```python
from build123d import *

# Parameters (mm, degrees)
F1_DEPTH = 5


with BuildPart() as f1:
    # F0 (on Right) → F1 (new body)
    with BuildSketch(Plane.YZ):
        with BuildLine():
            Line((-17.5, 52), (-22.5, 52))
            Line((-22.5, 52), (-22.5, 47))
            Line((-22.5, 47), (-23.8, 47))
            ThreePointArc((-23.8, 47), (-32.285281, 43.485281), (-35.8, 35))
            Line((-35.8, 35), (-35.8, 26))
            Line((-35.8, 26), (-34.8, 26))
            ThreePointArc((-34.8, 26), (-29.850253, 28.050253), (-27.8, 33))
            Line((-27.8, 33), (-27.8, 33.8))
            ThreePointArc((-27.8, 33.8), (-27.741421, 33.941421), (-27.6, 34))
            Line((-27.6, 34), (-22.7, 34))
            ThreePointArc((-22.7, 34), (-22.558579, 33.941421), (-22.5, 33.8))
            Line((-22.5, 33.8), (-22.5, -1))
            Line((-22.5, -1), (-23.8, -1))
            ThreePointArc((-23.8, -1), (-32.285281, -4.514719), (-35.8, -13))
            Line((-35.8, -13), (-35.8, -22))
            Line((-35.8, -22), (-34.8, -22))
            ThreePointArc((-34.8, -22), (-29.850253, -19.949747), (-27.8, -15))
            Line((-27.8, -15), (-27.8, -14.2))
            ThreePointArc((-27.8, -14.2), (-27.741421, -14.058579), (-27.6, -14))
            Line((-27.6, -14), (-22.7, -14))
            ThreePointArc((-22.7, -14), (-22.558579, -14.058579), (-22.5, -14.2))
            Line((-22.5, -14.2), (-22.5, -52))
            Line((-22.5, -52), (-17.5, -52))
            Line((-17.5, -52), (-17.5, -57))
            Line((-17.5, -57), (-7.5, -57))
            Line((-7.5, -57), (-7.5, -52))
            Line((-7.5, -52), (7.5, -52))
            Line((7.5, -52), (7.5, -57))
            Line((7.5, -57), (17.5, -57))
            Line((17.5, -57), (17.5, -52))
            Line((17.5, -52), (22.5, -52))
            Line((22.5, -52), (22.5, -45))
            Line((22.5, -45), (27.5, -45))
            Line((27.5, -45), (27.5, -27))
            Line((27.5, -27), (22.5, -27))
            Line((22.5, -27), (22.5, 27))
            Line((22.5, 27), (27.5, 27))
            Line((27.5, 27), (27.5, 45))
            Line((27.5, 45), (22.5, 45))
            Line((22.5, 45), (22.5, 52))
            Line((22.5, 52), (17.5, 52))
            Line((17.5, 52), (17.5, 57))
            Line((17.5, 57), (7.5, 57))
            Line((7.5, 57), (7.5, 52))
            Line((7.5, 52), (-7.5, 52))
            Line((-7.5, 52), (-7.5, 57))
            Line((-7.5, 57), (-17.5, 57))
            Line((-17.5, 57), (-17.5, 52))
        make_face()
    extrude(amount=F1_DEPTH)


solid = f1.part
```
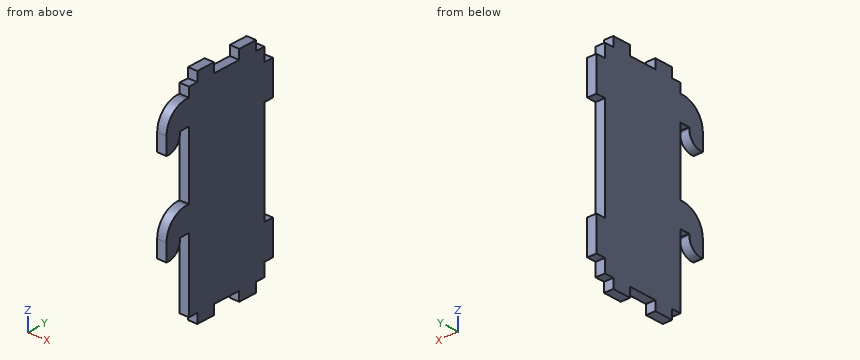
Work out the finished part from the listing and answer in its coordinate system (mm). Round coordinates to 2 decimals unless told otherwise and drop trailing zeros. Loops run counter-clockwise (first coordinate to the right, second up) from the corner with the lowest first, then second, coordinate; pieces in that order, holes last.
(1) Find the intervals of material crossed by L1, parallel to Y at x = 2.05, z = 52.5; L2, parallel to Z at x = 3.95, y = 3.5; L3, parallel to Y at x = 3.3, z = 3, in increasing order.
Computed values:
L1: y = -17.5 to -7.5, 7.5 to 17.5
L2: z = -52 to 52
L3: y = -22.5 to 22.5
(2) The part is cut by section C-C, the plane y = 4. Give the vertices of the cut face in (x, z).
Computed values:
outline: (0, -52) - (5, -52) - (5, 52) - (0, 52) - close
(3) Each of these flat-tipped pins is pushed along its axis until it touches: P1, Ø2.5, axis at x = 2, y = 24, coming from the +Z side; P2, Ø0.7, axis at x = 3.5, y = -23, coming from the +Z side; P3, Ø2.5, axis at x = 3.5, y = -21, coming from the -Z side. Where does it stop, or does it pass through?
Computed values:
P1: stops at z = 45
P2: stops at z = 47
P3: stops at z = -52
(4) The part is cut by section B-B, the plane z = -31. Give the vertices of the cut face in (x, y), and give its area (3 significant figures).
Computed values:
outline: (0, -22.5) - (5, -22.5) - (5, 27.5) - (0, 27.5) - close
area: 250 mm2
(5) The part is cut by section A-A, the plane y = -31.5. Give the vertices of the cut face in (x, z).
Computed values:
outline: (0, -21.17) - (5, -21.17) - (5, -3.8) - (0, -3.8) - close; (0, 26.83) - (5, 26.83) - (5, 44.2) - (0, 44.2) - close
